For this review, take the finished solid that the model builds, in its own axes (mm). Coordinates: 2 decimals unless noted, no trailing zeros. Write each loop counter-clockwise with the first axis right and the second up, starting at its lowest first coordinate (ties: lowest second). Pieces come first, ordered by that corner, then holes.
1) We need section A-A on y = 3.1. Write out the cut boundary in (x, z), then the cut area to 3 significant figures.
2) Insertion check: P1, Ø3, axis at x = -2.5, y = 1.5, coming from the +Z side. The pin has a flat end and moves straight along its axis. Give the tip position at first contact, or say it passes through.
3) We need section B-B on z = -218.5. Write out the cut boundary in (x, y), then the cut area to 3 significant figures.
4) To check wall thickness, follow line 1 along X through (y, z) = (1.4, -119.5); line 2 along X through (y, z) = (3, -152); line 3 along X through (y, z) = (3.7, -155). State the ranges of each line that lie inside material, in increasing order.
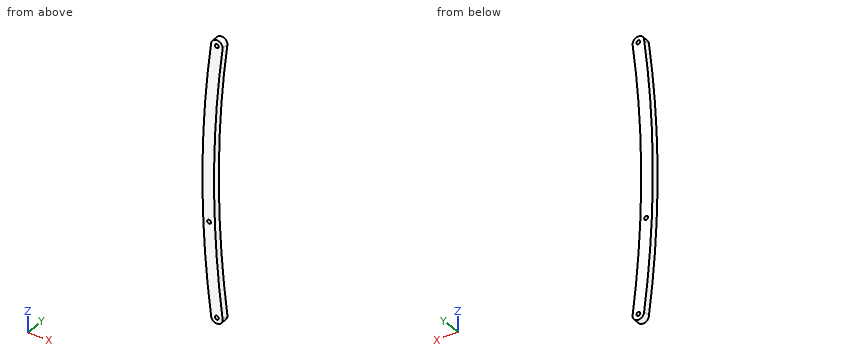
Autodesk Inventor part; units mm, degrees
ref_plane "YZ Plane" through (0, 0, 0) normal (1, 0, 0) x (0, 1, 0)
ref_plane "XZ Plane" through (0, 0, 0) normal (0, 1, 0) x (-1, 0, 0)
ref_plane "XY Plane" through (0, 0, 0) normal (0, 0, 1) x (1, 0, 0)
sketch "Sketch1" plane through (0, 0, 0) normal (0, 1, 0) x (-1, 0, 0)
  line L0 (0, 0) -> (0, -230.652) construction
  line L1 (5, 0) -> (5, -230.652)
  line L2 (-5, -230.652) -> (-5, 0)
  arc A0 (5, 0) -> (-5, 0) centre (0, 0) ccw
  arc A1 (-5, -230.652) -> (5, -230.652) centre (0, -230.652) ccw
  circle A2 centre (0, 0) radius 1.65
  circle A3 centre (0, -230.652) radius 1.65
  arc A4 (-5, -230.652) -> (-5, 0) centre (-897.5805, -115.326) ccw
  arc A5 (5, -230.652) -> (5, 0) centre (-887.5805, -115.326) ccw
  circle A6 centre (6.7073, -151.632) radius 1.65
  point P0 (0, -115.326)
  dimension "d0" = 3.3
  dimension "d1" = 3.3
  dimension "d2" = 10
  dimension "d3" = 230.652
  dimension "d14" = 900
  dimension "d15" = 900
  dimension "d16" = 3.3
  dimension "d17" = 79.02
extrude "Extrusion1" add sketch "Sketch1" along normal blind 6 contours A5 L1 | L1 A1 A4 A0
Result:
1. outline: (-5, -230.65) arc R5 ccw to (5, -230.65) arc R900 cw to (5, 0) arc R5 ccw to (-5, 0) arc R900 ccw to start; hole circle Ø3.3 at (-6.71, -151.63); hole circle Ø3.3 at (0, -230.65); hole circle Ø3.3 at (0, 0)
1. area: 2,360 mm2
2. P1: stops at z = 4.9
3. outline: (-6.49, 0) - (3.51, 0) - (3.51, 6) - (-6.49, 6) - close
3. area: 60.0 mm2
4. line 1: x = -12.41 to -2.41
4. line 2: x = -11.67 to -8.32, -5.1 to -1.67
4. line 3: x = -11.54 to -1.54
